from build123d import *

# Parameters (mm, degrees)
SKETCH_R        = 2.3
SKETCH_R_2      = 2.834
SKETCH_W        = 12
SKETCH_H        = 5.85
PAD_DEPTH       = 6
FILLET_R        = 1
CHAMFER_SIZE    = 0.4
CHAMFER001_SIZE = 0.3
FILLET001_R     = 1.8


with BuildPart() as part:
    # Sketch (on XY_Plane of Origin) → Pad (new body)
    with BuildSketch(Plane.XY):
        with BuildLine():
            Line((7, 15.5), (7, 3.055))
            Line((7, 3.055), (-7, 3.055))
            Line((-7, 3.055), (-7, 15.5))
            ThreePointArc((-7, 15.5), (-6.414214, 16.914214), (-5, 17.5))
            Line((-5, 17.5), (5, 17.5))
            ThreePointArc((5, 17.5), (6.414214, 16.914214), (7, 15.5))
        make_face()
        with Locations((-3, 13.5)):
            Circle(SKETCH_R, mode=Mode.SUBTRACT)
        with Locations((3.766, 13.5)):
            Circle(SKETCH_R_2, mode=Mode.SUBTRACT)
        with Locations((0, 6.98)):
            Rectangle(SKETCH_W, SKETCH_H, mode=Mode.SUBTRACT)
    extrude(amount=PAD_DEPTH)

    # Fillet
    fillet_edges = [part.edges().sort_by_distance(p)[0] for p in [
        (6, 9.905, 3),
        (6, 4.055, 3),
        (-6, 9.905, 3),
        (-6, 4.055, 3),
    ]]
    fillet(fillet_edges, radius=FILLET_R)

    # Chamfer
    chamfer_edges = [part.edges().sort_by_distance(p)[0] for p in [
        (-5.3, 13.5, 0),
        (-5.3, 13.5, 6),
    ]]
    chamfer(chamfer_edges, length=CHAMFER_SIZE)

    # Chamfer001
    chamfer001_edges = [part.edges().sort_by_distance(p)[0] for p in [
        (0.932, 13.5, 6),
    ]]
    chamfer(chamfer001_edges, length=CHAMFER001_SIZE)

    # Fillet001
    fillet001_edges = [part.edges().sort_by_distance(p)[0] for p in [
        (-7, 3.055, 3),
        (7, 3.055, 3),
    ]]
    fillet(fillet001_edges, radius=FILLET001_R)


with BuildPart() as part_1:
    # Body placement: moved
    add(part.part.moved(Location((0, 0, 0.8))))


solid = part_1.part
Read the model definition and answer for the solid it produces. Units are mm, in the model's axes. A direction names the side the tool comes from. Round coordinates to 2 decimals unless told otherwise and drop trailing zeros. Loops run counter-clockwise (first coordinate to the right, second up) from the corner with the lowest first, then second, coordinate; pieces in that order, holes last. Notation, with made-up numbers: (33.25, 4.5) - (79.25, 4.5) arc R20 cw to (79.25, 9.5) - close; hole circle Ø8 at (65.25, 45). An arc over 180 degrees is marked (long way). One line per question, with ' | ' between items. Start each with the question number.
Q1. Section A-A on y = 7.5 is taken. Give the vertices of the cut face in (x, z), plus the area to 3 significant figures.
Q2. For faces 5 (the flat face through (-6, 7, 4)), 6 (the flat face through (-7, 10, 4)), determine the directions among +Z, -Z, +X, -X, +Y, -Y from which every point of the face is accessible in a straight line to the end or side of a thin tool.
Q3. Section B-B on x = -3 is taken. Give the vertices of the cut face in (y, z) (3 decimals).
Q4. Section D-D on z = 1.55 is taken. Give the vertices of the cut face in (x, y) (3 decimals).
Q5. For a pull along Y with two mould halves and no side action, classify faces 1 (the flat face through (0, 3.055, 4)), 2 (the cylindrical face through (6.47, 14.35, 3.61)), 3 (the cylindrical face through (-5.715, 4.356, 3.842)), 4 (the flat face through (0, 17.5, 4)) as +Y half, -Y half, draft (parallel to the pull), parting line (faces both ways), or undercut.
Q6. Find the intervals of material crossed by L1, parallel to X at y = 8, z = 4.2; L2, parallel to Y at x = -1.75, z = 3.7 (3 decimals); L3, parallel to Y at x = -3.5, z = 2.7 (3 decimals), in increasing order.
Q7. Section C-C on y = 13.5 is taken. Give the vertices of the cut face in (x, z), plus the area to 3 significant figures.
Established:
1) outline: (-7, 0.8) - (-6, 0.8) - (-6, 6.8) - (-7, 6.8) - close; (6, 0.8) - (7, 0.8) - (7, 6.8) - (6, 6.8) - close | area: 12.0 mm²
2) face 5: +Z, -Z | face 6: +Z, -Z, -X, +Y, -Y
3) outline: (3.055, 0.8) - (4.055, 0.8) - (4.055, 6.8) - (3.055, 6.8) - close; (9.905, 0.8) - (10.8, 0.8) - (11.2, 1.2) - (11.2, 6.4) - (10.8, 6.8) - (9.905, 6.8) - close; (15.8, 1.2) - (16.2, 0.8) - (17.5, 0.8) - (17.5, 6.8) - (16.2, 6.8) - (15.8, 6.4) - close
4) outline: (-7, 4.855) arc R1.8 ccw to (-5.2, 3.055) - (5.2, 3.055) arc R1.8 ccw to (7, 4.855) - (7, 15.5) arc R2 ccw to (5, 17.5) - (-5, 17.5) arc R2 ccw to (-7, 15.5) - close; hole (-6, 5.055) arc R1 ccw to (-5, 4.055) - (5, 4.055) arc R1 ccw to (6, 5.055) - (6, 8.905) arc R1 ccw to (5, 9.905) - (-5, 9.905) arc R1 ccw to (-6, 8.905) - close; hole circle Ø4.6 at (-3, 13.5); hole circle Ø5.668 at (3.766, 13.5)
5) face 1: -Y half | face 2: undercut | face 3: undercut | face 4: +Y half
6) L1: -7 to -6, 6 to 7 | L2: 3.055 to 4.055, 9.905 to 11.569, 15.431 to 17.5 | L3: 3.055 to 4.055, 9.905 to 11.255, 15.745 to 17.5
7) outline: (-7, 0.8) - (-5.7, 0.8) - (-5.3, 1.2) - (-5.3, 6.4) - (-5.7, 6.8) - (-7, 6.8) - close; (-0.7, 1.2) - (-0.3, 0.8) - (0.93, 0.8) - (0.93, 6.5) - (0.63, 6.8) - (-0.3, 6.8) - (-0.7, 6.4) - close; (6.6, 0.8) - (7, 0.8) - (7, 6.8) - (6.9, 6.8) - (6.6, 6.5) - close | area: 22.0 mm²
